For this review, take the finished solid that the model builds, in its own axes (mm). Face numbers are marked on the shaded views. A direction names the side the tool comes from. Round coordinates to 2 decimals unless told otherwise and drop trailing zeros. Loops run counter-clockwise (first coordinate to the right, second up) from the corner with the lowest first, then second, coordinate; pieces in that order, holes last.
1. To check wall thickness, follow line 1 along Z through (x, y) = (20.5, 20.5); line 2 along Z through (x, y) = (54, -1); line 3 along Y through (x, z) = (60, -11). State the ranges of each line that lie inside material, in increasing order.
2. Consider section B-B on x = 41.5. State the section outline as (y, z) points, then the cut area to 3 significant figures.
3. Consider section A-A on y = 15. State the section outline as (x, z) points, then the cut area to 3 significant figures.
4. Draft analysis for pull direction Z (two halves, no side actions). For the marked faces 3, 4, 5 and 6, state which applies: released by +Z, released by -Z, zero draft, split by the parting line, or undercut.
5. Clearance check with flat-ended pins moving along their axes: pin 1 Ø7.5 at (x, z) = (39.5, 0) entering from +Y; pin 2 Ø14.5 at (y, z) = (-6.74, 3.92) entering from +X; pin 3 Ø3 at (y, z) = (18, -11) entering from +X. State where each tip first meets the part, or that it passes through.
6. Tool access review of the marked faces 1 and 2: name each direction out of +Z, -Z, +X, -X, +Y, -Y from which nothing blocks a thin tool from reaching the whole face with its end or side.
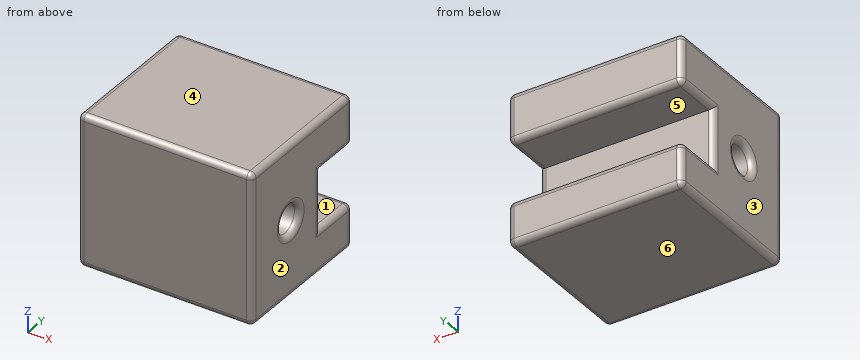
from build123d import *

# Parameters (mm, degrees)
F0_W     = 66.04
F0_H     = 66.04
F2_DEPTH = 76.2
F1_W     = 38.1
F1_H     = 25.4
F3_DEPTH = 76.2
F4_R     = 6.35
F5_DEPTH = 101.6
F6_R     = 2.54


with BuildPart() as f2:
    # F0 (on Right) → F2 (new body)
    with BuildSketch(Plane.YZ):
        with Locations((0.8847024292, 3.9172693067)):
            Rectangle(F0_W, F0_H)
    extrude(amount=F2_DEPTH)

    # F1 (on Right) → F3 (cut)
    with BuildSketch(Plane.YZ):
        with Locations((31.75, 2.6490623131)):
            Rectangle(F1_W, F1_H)
    extrude(amount=F3_DEPTH, mode=Mode.SUBTRACT)

    # F4 (on face) → F5 (cut)
    with BuildSketch(Plane.YZ.offset(76.2)):
        with Locations((-6.7352975708, 3.9172693067)):
            Circle(F4_R)
    extrude(amount=-F5_DEPTH, mode=Mode.SUBTRACT)

    # F6
    f6_edges = [f2.edges().sort_by_distance(p)[0] for p in [
        (0, 33.904702, 26.143166),
        (0, 0.884702, 36.937269),
        (0, 0.884702, -29.102731),
        (0, -32.135298, 3.917269),
        (0, 33.904702, -19.576834),
        (0, 23.302351, -10.050938),
        (0, 12.7, 2.649062),
        (0, 23.302351, 15.349062),
        (0, -13.085298, 3.917269),
        (76.2, 0.884702, -29.102731),
        (76.2, -32.135298, 3.917269),
        (76.2, 33.904702, -19.576834),
        (76.2, 0.884702, 36.937269),
        (76.2, 23.302351, -10.050938),
        (76.2, 33.904702, 26.143166),
        (76.2, 12.7, 2.649062),
        (76.2, 23.302351, 15.349062),
        (76.2, -13.085298, 3.917269),
        (38.1, 33.904702, 36.937269),
        (38.1, 33.904702, 15.349062),
        (38.1, 33.904702, -10.050938),
        (38.1, 33.904702, -29.102731),
        (38.1, -32.135298, -29.102731),
        (38.1, -32.135298, 36.937269),
    ]]
    fillet(f6_edges, radius=F6_R)


solid = f2.part
Resolved:
1. line 1: z = -29.1 to -10.05, 15.35 to 36.94
1. line 2: z = -29.1 to 1.19, 6.64 to 36.94
1. line 3: y = -32.14 to 33.34
2. outline: (-32.14, -26.56) arc R2.54 ccw to (-29.6, -29.1) - (31.36, -29.1) arc R2.54 ccw to (33.9, -26.56) - (33.9, -12.59) arc R2.54 ccw to (31.36, -10.05) - (12.7, -10.05) - (12.7, 15.35) - (31.36, 15.35) arc R2.54 ccw to (33.9, 17.89) - (33.9, 34.4) arc R2.54 ccw to (31.36, 36.94) - (-29.6, 36.94) arc R2.54 ccw to (-32.14, 34.4) - close; hole circle Ø12.7 at (-6.74, 3.92)
2. area: 3,690 mm2
3. outline: (0, -26.56) arc R2.54 ccw to (2.54, -29.1) - (73.66, -29.1) arc R2.54 ccw to (76.2, -26.56) - (76.2, -12.59) arc R2.54 ccw to (73.66, -10.05) - (2.54, -10.05) arc R2.54 ccw to (0, -12.59) - close; (0, 17.89) arc R2.54 ccw to (2.54, 15.35) - (73.66, 15.35) arc R2.54 ccw to (76.2, 17.89) - (76.2, 34.4) arc R2.54 ccw to (73.66, 36.94) - (2.54, 36.94) arc R2.54 ccw to (0, 34.4) - close
3. area: 3,090 mm2
4. face 3: zero draft
4. face 4: released by +Z
4. face 5: undercut
4. face 6: released by -Z
5. pin 1: stops at y = 12.7
5. pin 2: stops at x = 75.6
5. pin 3: stops at x = 76.2
6. face 1: +X, -X, +Y
6. face 2: +Z, -Z, +X, +Y, -Y
